Part model, mm, in its own coordinate system. A direction names the side the tool comes from. Round coordinates to 2 decimals unless told otherwise and drop trailing zeros. Write each loop counter-clockwise with the first axis right and the second up, starting at its lowest first coordinate (ties: lowest second). Pieces come first, ordered by that corner, then holes. Notation, with made-up numbers: (1.5, 57) -> (37.5, 57) arc R26 cw to (37.5, 90) -> close; hole circle Ø8 at (-30.75, -21.75). An arc over 180 degrees is marked (long way). Return JSON: item names as keys, results as strings. Group by question number.
(1) Drop flat-ended pins along their axis: pin 1 Ø3.5 at (x, y) = (7, -3) entering from +Z; pin 2 Ø1 at (y, z) = (9, 3.5) entering from +X; pin 3 Ø0.8 at (x, z) = (0.5, 5.5) entering from -Y. Give the stop position or say it passes through.
(2) Tool access for faces 1 (the flat face through (-6, 0, 5)), 2 (the flat face through (0, -12.46, 5.4)), 3 (the flat face through (5, 0, 5)), 4 (the cylindrical face through (11.923, 3.755, 2.465)): list every direction of +Z, -Z, +X, -X, +Y, -Y with a clear straight run to the whole face (end or side of a thin tool).
(3) Mould opens along Z. For faces 5 (the flat face through (0, 12.46, 5.4)), 6 (the cylindrical face through (0.715, 0.174, 5.699)), 7 (the flat face through (0, 0, 0)) say: +Z half, -Z half, draft (parallel to the pull), parting line (faces both ways), or undercut.
(4) Saw through at B-B (z = 3). List the corners of the cut face in (x, y), plus the area to 3 significant figures.
(5) Saw through at C-C (x = -3). List the corners of the cut face in (y, z).
(6) Drill centre lines: L1, parallel to Z at x = -6.5, y = -2.25; L2, parallel to X at y = 9.25, z = 0.75; L3, parallel to X at y = 3, z = 4.75. Where is each one in solid material? Low to high. Write a range as from..to.
from build123d import *

# Parameters (mm, degrees)
F0_R     = 12.5
F1_DEPTH = 5
F2_W     = 2
F2_H     = 24.9198715888
F3_DEPTH = 1
F4_R     = 0.99999


# Not quite as in the source:
# - a fillet or chamfer is up to 0.001 mm smaller than in the source, because OpenCascade refuses the exact size


with BuildPart() as f1:
    # F0 (on Top) → F1 (new body)
    with BuildSketch(Plane.XY):
        Circle(F0_R)
    extrude(amount=F1_DEPTH)

    # F2 (on face) → F3 (join)
    with BuildSketch(Plane.XY.offset(5)):
        Rectangle(F2_W, F2_H)
    extrude(amount=F3_DEPTH)

    # F4 (radius 1 in the source; OpenCascade refuses exactly that, so slightly less here)
    f4_edges = [f1.edges().sort_by_distance(p)[0] for p in [
        (1, 0, 6),
        (-1, 0, 6),
    ]]
    fillet(f4_edges, radius=F4_R)


solid = f1.part
Computed values:
{
 "1": {"pin 1": "z = 5", "pin 2": "x = 9.17", "pin 3": "y = -12.46"},
 "2": {"face 1": "+Z, -X, +Y, -Y", "face 2": "+Z, +X, -X, -Y", "face 3": "+Z, +X, +Y, -Y", "face 4": "+Z, -Z"},
 "3": {"face 5": "draft", "face 6": "+Z half", "face 7": "-Z half"},
 "4": {"outline": "circle Ø25 at (0, 0)", "area": "491 mm2"},
 "5": {"outline": "(-12.13, 0) -> (12.13, 0) -> (12.13, 5) -> (-12.13, 5) -> close"},
 "6": {"L1": "0..5", "L2": "-8.41..8.41", "L3": "-12.13..12.13"}
}
